```python
from build123d import *

# Parameters (mm, degrees)
F0_W     = 209.55
F0_H     = 381
F1_DEPTH = 6.35
F2_W     = 50.8
F2_H     = 254
F3_DEPTH = 25.4
F4_D     = 3.175
F4_DEPTH = 19.05


with BuildPart() as f1:
    # F0 (on Top) → F1 (new body)
    with BuildSketch(Plane.XY):
        Rectangle(F0_W, F0_H)
    extrude(amount=F1_DEPTH)

    # F2 (on face) → F3 (cut)
    with BuildSketch(Plane.XY.offset(6.35)):
        with Locations((50.8, 0)):
            Rectangle(F2_W, F2_H)
    extrude(amount=-F3_DEPTH, mode=Mode.SUBTRACT)

    # F4
    with Locations(Plane.XY.offset(6.35)):
        with Locations((0, -104.775), (0, -85.725), (0, 85.725), (0, 104.775)):
            Hole(F4_D / 2, depth=F4_DEPTH)


solid = f1.part
```
The model under review builds one solid part; all positions refer to its coordinate system, in mm. Round coordinates to 2 decimals unless told otherwise and drop trailing zeros. Loops run counter-clockwise (first coordinate to the right, second up) from the corner with the lowest first, then second, coordinate; pieces in that order, holes last. Notation, with made-up numbers: (-19, 8) - (16, 8) arc R23 ccw to (16, 19) - close; hole circle Ø4 at (80, -7). An arc over 180 degrees is marked (long way). Use a Markdown table: item, result. Add a question column.
Q1. For probe 1 along Y at (x, z) = (0, 1.75); probe 2 along X at (y, z) = (-53, 0.5) (3 decimals); probe 3 along Y at (x, z) = (47.5, 5.5), list the stretches that pass through material, from the lowest coordinate up.
Q2. Add section A-A (x = 30). State the section outline as (y, z) points, plus the area to 3 significant figures.
Q3. Add section C-C (z = 4.5). State the section outline as (x, y) points (1 decimal), plus the area to 3 significant figures.
Q4. Add section B-B (y = 115). State the section outline as (x, z) points (3 decimals), plus the area to 3 significant figures.
Q5. Insertion check: pin 1 Ø2.5 at (x, y) = (0, 104.775) entering from -Z; pin 2 Ø4 at (x, y) = (0, -104.775) entering from -Z. Each pin has a flat end and moves straight along its axis. Give the tip position at first contact, or say it passes through.
Worked answers:
| question | item | result |
|---|---|---|
| 1 | probe 1 | -190.5 to -106.36, -103.19 to -87.31, -84.14 to 84.14, 87.31 to 103.19, 106.36 to 190.5 |
| 1 | probe 2 | -104.775 to 25.4, 76.2 to 104.775 |
| 1 | probe 3 | -190.5 to -127, 127 to 190.5 |
| 2 | outline | (-190.5, 0) - (-127, 0) - (-127, 6.35) - (-190.5, 6.35) - close; (127, 0) - (190.5, 0) - (190.5, 6.35) - (127, 6.35) - close |
| 2 | area | 806 mm² |
| 3 | outline | (-104.8, -190.5) - (104.8, -190.5) - (104.8, 190.5) - (-104.8, 190.5) - close; hole circle Ø3.2 at (0, -104.8); hole circle Ø3.2 at (0, -85.7); hole circle Ø3.2 at (0, 85.7); hole circle Ø3.2 at (0, 104.8); hole (25.4, -127) - (76.2, -127) - (76.2, 127) - (25.4, 127) - close |
| 3 | area | 66,900 mm² |
| 4 | outline | (-104.775, 0) - (25.4, 0) - (25.4, 6.35) - (-104.775, 6.35) - close; (76.2, 0) - (104.775, 0) - (104.775, 6.35) - (76.2, 6.35) - close |
| 4 | area | 1,010 mm² |
| 5 | pin 1 | through |
| 5 | pin 2 | z = 0 |
